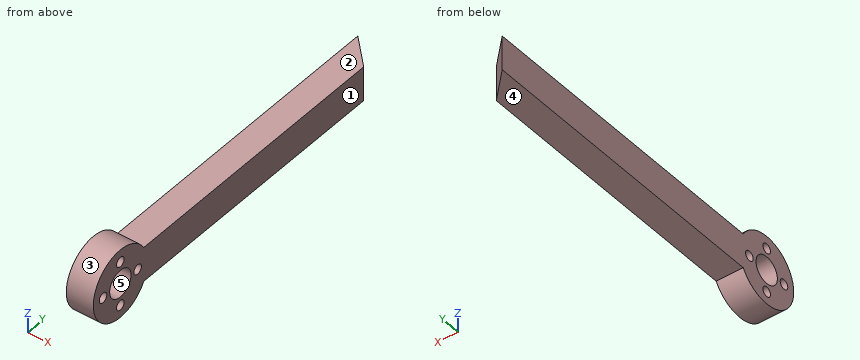
from build123d import *

# Parameters (mm, degrees)
SKETCH1_R           = 5.0165
SKETCH1_R_2         = 1.778
BOSS_EXTRUDE1_DEPTH = 9.906
BOSS_EXTRUDE2_DEPTH = 12.7


with BuildPart() as part:
    # Sketch1 → Boss-Extrude1 (new body)
    with BuildSketch(Plane(origin=(0, 0, 0), x_dir=(0, 0, -1), z_dir=(1, 0, 0))):
        with BuildLine():
            Line((-6.35, -50.8), (-6.35, 52.501477372))
            Line((-6.35, 52.501477372), (6.35, 52.501477372))
            Line((6.35, 52.501477372), (6.35, -50.8))
            ThreePointArc((6.35, -50.8), (0, -74.498522628), (-6.35, -50.8))
        make_face()
        with Locations((0, -61.798522628)):
            Circle(SKETCH1_R, mode=Mode.SUBTRACT)
        with Locations((-8.128, -61.798522628)):
            Circle(SKETCH1_R_2, mode=Mode.SUBTRACT)
        with Locations((8.128, -61.798522628)):
            Circle(SKETCH1_R_2, mode=Mode.SUBTRACT)
        with Locations((0, -53.670522628)):
            Circle(SKETCH1_R_2, mode=Mode.SUBTRACT)
        with Locations((0, -69.926522628)):
            Circle(SKETCH1_R_2, mode=Mode.SUBTRACT)
    extrude(amount=BOSS_EXTRUDE1_DEPTH)

    # Sketch2 → Boss-Extrude2 (add)
    with BuildSketch(Plane.XY.offset(6.35)):
        Polygon((9.906, 52.501477372), (0, 52.501477372), (0, 62.407477372), align=None)
    extrude(amount=-BOSS_EXTRUDE2_DEPTH)


solid = part.part
Part model, mm, in its own coordinate system. Face numbers are marked on the shaded views. A direction names the side the tool comes from. Give positions to 0.01 mm unless a question says otherwise; leave off trailing zeros. Order: outer loops, then holes, each group sorted by start corner. A loop starts at its lowest first (then second) coordinate and runs counter-clockwise, first axis right, second up. Notation, with made-up numbers: (-35, 18.5) - (10, 18.5) arc R23 ccw to (10, 39.5) - close; hole circle Ø11 at (8.25, -31). An arc over 180 degrees is marked (long way). Use a Markdown table: item, result.
1) Saw through at B-B on x = 6. List the corners of the cut face in (y, z).
Checked values:
| item | result |
|---|---|
| outline | (-50.8, -6.35) - (56.41, -6.35) - (56.41, 6.35) - (-50.8, 6.35) arc R12.7 ccw (long way) to start; hole circle Ø3.56 at (-69.93, 0); hole circle Ø10.03 at (-61.8, 0); hole circle Ø3.56 at (-61.8, -8.13); hole circle Ø3.56 at (-61.8, 8.13); hole circle Ø3.56 at (-53.67, 0) |
2) Probe L1, parallel to Z at x = 1.75, y = -19.5; L2, parallel to Y at x = 4.75, z = 0.5. List the from-to ranges inside material, lowest first. Write a range as from..to.
Checked values:
| item | result |
|---|---|
| L1 | -6.35..6.35 |
| L2 | -74.49..-71.63, -68.22..-66.79, -56.81..-55.38, -51.96..57.66 |
3) 3-axis set-ups, long thin cutter, end or side, ignore diameter. For the marked faces 1 and 2: which of +Z, -Z, +X, -X, +Y, -Y reach the whole face in a straight line?
Checked values:
| item | result |
|---|---|
| face 1 | +Z, -Z, +X, +Y, -Y |
| face 2 | +Z, +X, -X, +Y |
4) Flat gauge pins, fed straight in: P1, Ø5, axis at x = 4.5, y = -34, coming from the +Z side; P2, Ø10, axis at y = -22.5, z = 6.5, coming from the -X side; P3, Ø2, axis at x = 7, z = 3, coming from the +Y side; P4, Ø1.5, axis at x = 9, z = -4.5, coming from the +Y side. Where does each tip first touch, or does it go through?
Checked values:
| item | result |
|---|---|
| P1 | z = 6.35 |
| P2 | x = 0 |
| P3 | y = 56.41 |
| P4 | y = 54.16 |
5) Saw through at C-C on y = 6.5. List the corners of the cut face in (x, z), plus the area to 3 significant figures.
Checked values:
| item | result |
|---|---|
| outline | (0, -6.35) - (9.91, -6.35) - (9.91, 6.35) - (0, 6.35) - close |
| area | 126 mm² |
6) Saw through at A-A on z = 0. List the corners of the cut face in (x, y).
Checked values:
| item | result |
|---|---|
| outline | (0, -74.5) - (9.91, -74.5) - (9.91, -71.7) - (0, -71.7) - close; (0, -68.15) - (9.91, -68.15) - (9.91, -66.82) - (0, -66.82) - close; (0, -56.78) - (9.91, -56.78) - (9.91, -55.45) - (0, -55.45) - close; (0, -51.89) - (9.91, -51.89) - (9.91, 52.5) - (0, 62.41) - close |
7) Two-plate mould, pull along Y, no slides. Class the marked faces 3, 4 and 5: +Y half, -Y half, draft (parallel to the pull), parting line (faces both ways), or undercut.
Checked values:
| item | result |
|---|---|
| face 3 | parting line |
| face 4 | draft |
| face 5 | undercut |
